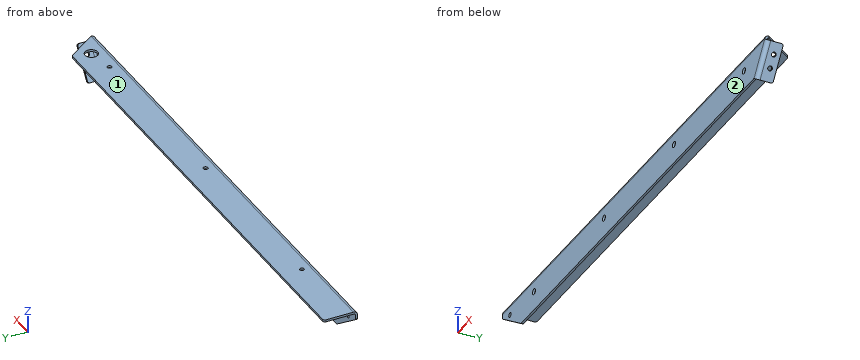
```python
from build123d import *

# Parameters (mm, degrees)
BASE_FLANGE1_DEPTH = 762
CUT_EXTRUDE1_DEPTH = 3.175
CUT_EXTRUDE2_DEPTH = 3.175
EDGE_FLANGE1_DEPTH = 54.26343047
SKETCH9_R          = 3.175
SKETCH9_R_2        = 9.525
SKETCH9_R_3        = 3.429
CUT_EXTRUDE3_DEPTH = 3.175
SKETCH10_R         = 4.3688
SKETCH10_R_2       = 3.429
CUT_EXTRUDE4_DEPTH = 4.9022
SKETCH11_R         = 3.429
CUT_EXTRUDE5_DEPTH = 3.175
FILLET1_R          = 3.175


# Sheet-metal steps are written as plain solids
with BuildPart() as part:
    # Sketch1 → Base-Flange1 (new body)
    with BuildSketch(Plane(origin=(0, 0, 0), x_dir=(0, 0, -1), z_dir=(1, 0, 0))):
        with BuildLine():
            Line((0, 50.8), (0, 6.35))
            ThreePointArc((0, 6.35), (1.859871939, 1.859871939), (6.35, 0))
            Line((6.35, 0), (50.8, 0))
            Line((50.8, 0), (50.8, 3.175))
            Line((50.8, 3.175), (6.35, 3.175))
            ThreePointArc((6.35, 3.175), (4.10493597, 4.10493597), (3.175, 6.35))
            Line((3.175, 6.35), (3.175, 50.8))
            Line((3.175, 50.8), (0, 50.8))
        make_face()
    extrude(amount=BASE_FLANGE1_DEPTH)

    # Sketch3 → Cut-Extrude1 (cut)
    with BuildSketch(Plane(origin=(0, 0, -3.175), x_dir=(-1, 0, 0), z_dir=(0, 0, -1))):
        Polygon((-762, 6.35), (-762, 50.8), (-730.875774927, 50.8), align=None)
    extrude(amount=-CUT_EXTRUDE1_DEPTH, mode=Mode.SUBTRACT)

    # Sketch4 → Cut-Extrude2 (cut)
    with BuildSketch(Plane(origin=(0, 3.175, 0), x_dir=(1, 0, 0), z_dir=(0, 1, 0))):
        Polygon((762, 6.35), (730.875774927, 50.8), (762, 50.8), align=None)
        Polygon((0, 12.7), (54.412439057, 50.8), (0, 50.8), align=None)
    extrude(amount=-CUT_EXTRUDE2_DEPTH, mode=Mode.SUBTRACT)

    # Edge-Flange1 section (across the edge) → Edge-Flange1 (add)
    with BuildSketch(Plane(origin=(764.600807741, 3.175, -8.171105185), x_dir=(-0.8191520442889946, 3.4914813388431337e-15, 0.5735764363510422), z_dir=(-0.5735764363510422, 0, -0.8191520442889946))):
        with BuildLine():
            Line((-3.175, 3.175), (-3.175, 22.225))
            Line((-3.175, 22.225), (0, 22.225))
            Line((0, 22.225), (0, 3.175))
            ThreePointArc((0, 3.175), (0.92993597, 0.92993597), (3.175, 0))
            Line((3.175, 0), (3.175, -3.175))
            ThreePointArc((3.175, -3.175), (-1.315128061, -1.315128061), (-3.175, 3.175))
        make_face()
    extrude(amount=EDGE_FLANGE1_DEPTH)

    # Sketch9 → Cut-Extrude3 (cut)
    with BuildSketch(Plane.XY):
        with Locations((124.841, 19.05)):
            Circle(SKETCH9_R)
        with Locations((683.641, 19.05)):
            Circle(SKETCH9_R)
        with Locations((723.9, 25.4)):
            Circle(SKETCH9_R_2)
        with Locations((404.241, 19.05)):
            Circle(SKETCH9_R_3)
    extrude(amount=-CUT_EXTRUDE3_DEPTH, mode=Mode.SUBTRACT)

    # Sketch10 → Cut-Extrude4 (cut)
    with BuildSketch(Plane.XZ):
        with Locations(Location((92.075, -22.225, 0), (0, 0, 270))):
            Circle(SKETCH10_R)
        with Locations(Location((295.275, -22.225, 0), (0, 0, 270))):
            Circle(SKETCH10_R)
        with Locations(Location((498.475, -22.225, 0), (0, 0, 270))):
            Circle(SKETCH10_R)
        with Locations(Location((701.675, -22.225, 0), (0, 0, 270))):
            Circle(SKETCH10_R)
        with Locations(Location((22.225, -19.05, 0), (0, 0, 270))):
            Circle(SKETCH10_R_2)
    extrude(amount=-CUT_EXTRUDE4_DEPTH, mode=Mode.SUBTRACT)

    # Sketch11 → Cut-Extrude5 (cut)
    with BuildSketch(Plane(origin=(519.494814159, 0, -363.754184935), x_dir=(-0.5735764363510422, 1.0031284501279259e-15, -0.8191520442889946), z_dir=(0.8191520442889947, -1.4326158965565184e-15, -0.5735764363510422))):
        with Locations((-396.015198548, 15.875)):
            Circle(SKETCH11_R)
        with Locations((-415.065198548, 15.875)):
            Circle(SKETCH11_R)
    extrude(amount=-CUT_EXTRUDE5_DEPTH, mode=Mode.SUBTRACT)

    # Fillet1
    fillet1_edges = [part.edges().sort_by_distance(p)[0] for p in [
        (730.875774927, 50.8, -1.5875),
        (0, 1.5875, -12.7),
        (54.412439057, 1.5875, -50.8),
        (765.901211611, 25.4, -9.081657778),
        (734.776986538, 25.4, -53.531657778),
        (0, 50.8, -1.5875),
    ]]
    fillet(fillet1_edges, radius=FILLET1_R)


solid = part.part
```
Geometry: final body of the model. Coordinates: model frame, mm. Face numbers are marked on the shaded views. Round coordinates to 2 decimals unless told otherwise and drop trailing zeros. Write each loop counter-clockwise with the first axis right and the second up, starting at its lowest first coordinate (ties: lowest second). Pieces come first, ordered by that corner, then holes. Notation, with made-up numbers: M 57,-19 L 116,-19 A11 ccw 116,-9 Z; hole C 20,73 d7. An arc over 180 degrees is marked long. Answer in a Markdown table with one row per item. Add a question column.
(1) Cut plane A-A, the plane x = 469. Return the cut outline in (y, z) (3 decimals), then the cut area to 3 significant figures.
(2) Contact query for flat-ended pins moving along their axis: pin 1 (8 mm diameter, centred on x = 701.675, z = -22.225, fed in from +Y); pin 2 (1.6 mm diameter, centred on x = 226.5, y = 2, fed in from -Z); pin 3 (4 mm diameter, centred on x = 662.5, y = 26, fed in from -Z) (3 decimals); pin 4 (9 mm diameter, centred on x = 404.241, y = 19.05, fed in from +Z). Output: stop coordinate, or through.
(3) Ray query, L1, parallel to Y at x = 723.9, z = -2.3 (3 decimals); L2, parallel to Y at x = 42, z = -20.5 (3 decimals); L3, parallel to Z at x = 719.5, y = 34.5 (3 decimals). Return the intervals inside material, ascending.
(4) Draft query along Z for the marked faces 1 and 2. Return one class per face: pulls with the +Z half, pulls with the -Z half, needs draft (parallel to the pull), parting line crosses it, or undercut.
Established:
| question | item | result |
|---|---|---|
| 1 | outline | M 0,-50.8 L 3.175,-50.8 L 3.175,-6.35 A3.175 cw 6.35,-3.175 L 50.8,-3.175 L 50.8,0 L 6.35,0 A6.35 ccw 0,-6.35 Z |
| 1 | area | 306 mm² |
| 2 | pin 1 | through |
| 2 | pin 2 | z = -50.8 |
| 2 | pin 3 | z = -3.175 |
| 2 | pin 4 | z = 0 |
| 3 | L1 | 1.459 to 15.875, 34.925 to 50.8 |
| 3 | L2 | 0 to 3.175 |
| 3 | L3 | -3.175 to 0 |
| 4 | face 1 | pulls with the +Z half |
| 4 | face 2 | needs draft |
